Autodesk Fusion 360 part; units mm, degrees
sketch "Sketch1" plane through (0, 0, 0) normal (0, 0, 1) x (1, 0, 0)
  circle A0 centre (0, 0) radius 2.5
  circle A1 centre (0, 0) radius 1.75
  dimension "d1" = 5
  dimension "d2" = 3.5
extrude "Extrude1" add sketch "Sketch1" along normal blind 4 contours A0 | A1
extrude "Extrude2" add sketch "Sketch1" along normal blind 7 contours A1
fillet "Fillet1" radius 1 1 edges at (-2.3308, -0.904, 0)
Verification items for the finished model (mm, model axes). A direction names the side the tool comes from. Give positions to 0.01 mm unless a question says otherwise; leave off trailing zeros. Loops run counter-clockwise (first coordinate to the right, second up) from the corner with the lowest first, then second, coordinate; pieces in that order, holes last. Notation, with made-up numbers: M 3.5,69 L 44.5,69 A22 ccw 44.5,85 Z; hole C 77.5,-17 d5. An arc over 180 degrees is marked long. One line per question, with ' | ' between items.
Item 1: Section check A-A, the plane x = 0. Record the cut outline in (y, z), plus the area to 3 significant figures.
Completed:
outline: M -2.5,1 A1 ccw -1.5,0 L 1.5,0 A1 ccw 2.5,1 L 2.5,4 L 1.75,4 L 1.75,7 L -1.75,7 L -1.75,4 L -2.5,4 Z | area: 30.1 mm^2
Item 2: Section check C-C, the plane z = 1.5. Record the cut outline in (x, y), plus the area to 3 significant figures.
Completed:
outline: C 0,0 d5 | area: 19.6 mm^2
Item 3: Section check D-D, the plane z = 5.75. Record the cut outline in (x, y), plus the area to 3 significant figures.
Completed:
outline: C 0,0 d3.5 | area: 9.62 mm^2
Item 4: Thickness scan on line 1 (Y direction, x = -1.75, z = 3.5); line 2 (X direction, y = 0.3, z = 2); line 3 (Y direction, x = -1.4, z = 6.25). Record the ranges inside material, lowest first. Write a range as [from, to].
Completed:
line 1: y = [-1.79, 1.79] | line 2: x = [-2.48, 2.48] | line 3: y = [-1.05, 1.05]
Item 5: Tool access check on faces 1 (the face through (1, 2, 4)), 2 (the face through (-0.54, 2.44, 2.48)). Record the directions out of +Z, -Z, +X, -X, +Y, -Y that give a thin tool (end or side, any length) a straight path to the whole face; none if there is none.
Completed:
face 1: +Z | face 2: +Z, -Z
Item 6: Depth check by flat-ended pin: P1, Ø1, axis at x = 1.5, z = 2, coming from the +Y side. Enter the tip coordinate at first touch or a pass-through.
Completed:
P1: stops at y = 2.29
